```python
from build123d import *

# Parameters (mm, degrees)
F0_R     = 7.5
F0_R_2   = 4
F2_DEPTH = 15
F3_R     = 6
F4_DEPTH = 9
F5_SIZE  = 1.99999


# Not quite as in the source:
# - a fillet or chamfer is up to 0.001 mm smaller than in the source, because OpenCascade refuses the exact size


with BuildPart() as f2:
    # F0 (on Top) → F2 (new body)
    with BuildSketch(Plane.XY):
        Circle(F0_R)
        Circle(F0_R_2, mode=Mode.SUBTRACT)
    extrude(amount=-F2_DEPTH)

    # F3 (on offset) → F4 (cut)
    with BuildSketch(Plane.XY.offset(-3)):
        Circle(F3_R)
    extrude(amount=-F4_DEPTH, mode=Mode.SUBTRACT)

    # F5 (size 2 in the source; OpenCascade refuses exactly that, so slightly less here)
    f5_edges = [f2.edges().sort_by_distance(p)[0] for p in [
        (-4, 0, -3),
        (-4, 0, -12),
    ]]
    chamfer(f5_edges, length=F5_SIZE)


solid = f2.part
```
The listing builds one solid part. Answer for the finished solid, in the listing's coordinates (mm). A direction names the side the tool comes from. Coordinates: 2 decimals unless noted, no trailing zeros. Loops run counter-clockwise (first coordinate to the right, second up) from the corner with the lowest first, then second, coordinate; pieces in that order, holes last. Notation, with made-up numbers: (13, 30.25) - (25, 30.25) arc R17 ccw to (25, 45.25) - close; hole circle Ø11 at (29.25, 22). An arc over 180 degrees is marked (long way). Use a Markdown table: item, result. Add a question column.
1) The part is cut by section C-C, the plane z = -11. Give the vertices of the cut face in (x, y).
2) For faces 1 (the conical face through (3.935, 1.239, -13.875)), 2 (the cylindrical face through (-0.867, -3.905, -14.493)), determine the directions among +Z, -Z, +X, -X, +Y, -Y from which every point of the face is accessible in a straight line to the end or side of a thin tool.
3) The part is cut by section D-D, the plane z = -1.75. Give the vertices of the cut face in (x, y).
4) The mould has two halves that part along X. Classify faces 3 (the flat face through (3, -3, -15)), 4 (the cylindrical face through (-7.493, 0.33, -7.395)), 5 (the cylindrical face through (-0.867, -3.905, -0.493)), 6 (the conical face through (3.935, 1.239, -1.125)): released by +X, released by -X, zero draft, split by the parting line, or undercut.
5) Find the intervals of material crossed by line 1 (Y direction, x = 0, z = -0.55); line 2 (X direction, y = -4.25, z = -11.5); line 3 (Y direction, x = 0, z = -6.25), in increasing order.
6) Given pin 1 (3.5 mm diameter, centred on x = 1, y = 1, fed in from -Z); pin 2 (5 mm diameter, centred on x = -4.5, z = -2, fed in from -Y); pin 3 (2 mm diameter, centred on x = 3.5, z = -13, fed in from +Y); pin 4 (3.5 mm diameter, centred on x = 2.5, y = -2.5, fed in from +Z), each flat-ended and moving along its own axis, determine where each tip first touches the part or whether it passes through.
Here are the results:
| question | item | result |
|---|---|---|
| 1 | outline | circle Ø15 at (0, 0); hole circle Ø12 at (0, 0) |
| 2 | face 1 | none |
| 2 | face 2 | +Z, -Z |
| 3 | outline | circle Ø15 at (0, 0); hole circle Ø9.5 at (0, 0) |
| 4 | face 3 | zero draft |
| 4 | face 4 | split by the parting line |
| 4 | face 5 | undercut |
| 4 | face 6 | undercut |
| 5 | line 1 | y = -7.5 to -4, 4 to 7.5 |
| 5 | line 2 | x = -6.18 to -4.24, 4.24 to 6.18 |
| 5 | line 3 | y = -7.5 to -6, 6 to 7.5 |
| 6 | pin 1 | passes through |
| 6 | pin 2 | stops at y = -7.23 |
| 6 | pin 3 | stops at y = 7.07 |
| 6 | pin 4 | stops at z = 0 |
